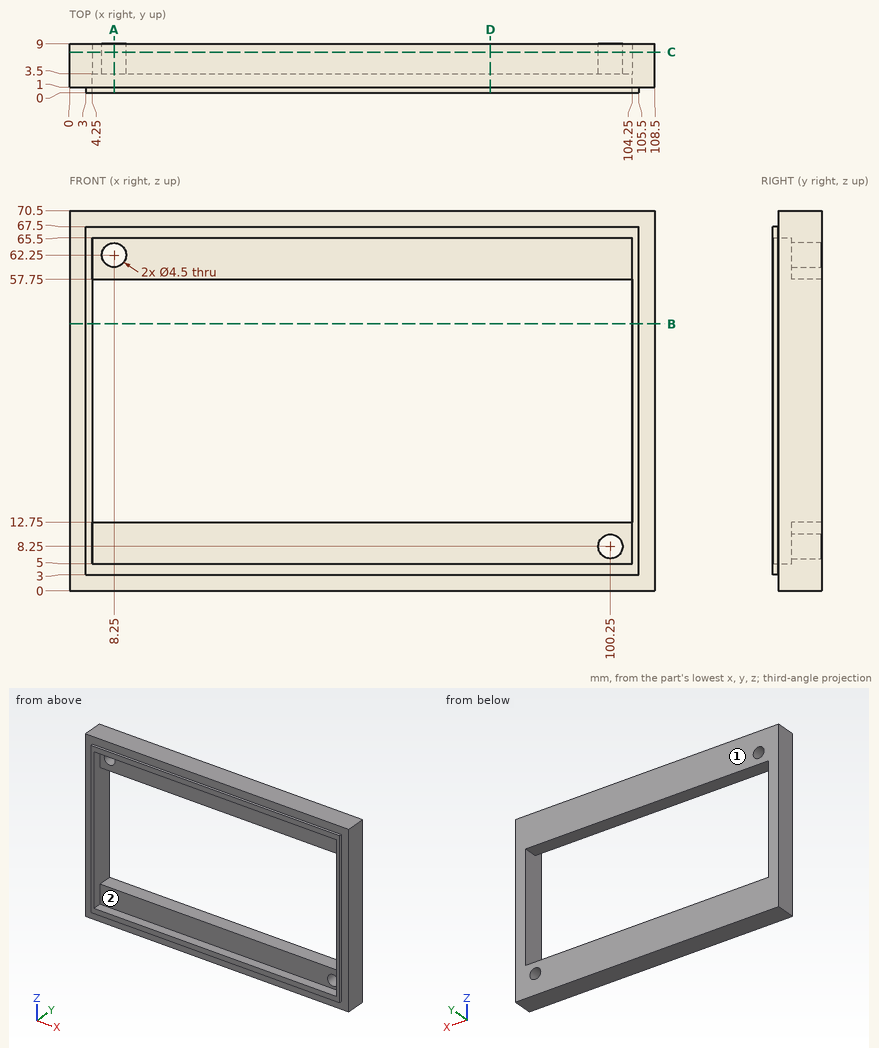
The figure shows three views and two pictorial views of one solid part (mm, origin at its lowest corner). Answer the questions. Coordinates: 2 decimals unless noted, no trailing zeros. Order: outer loops, then holes, each group sorted by start corner. A loop starts at its lowest first (then second) coordinate and runs counter-clockwise, first axis right, second up. Notation, with made-up numbers: (2.25, 30.5) - (44.25, 30.5) arc R30 cw to (44.25, 56.5) - close; hole circle Ø10 at (20, 14). An arc over 180 degrees is marked (long way). Answer as a JSON object with one key per item and string values.
1. Find section D-D on x = 78. Determine the outline of the cut face in (y, z).
Output values:
{"outline": "(0, 3) - (1, 3) - (1, 0) - (9, 0) - (9, 12.75) - (3.5, 12.75) - (3.5, 5) - (0, 5) - close; (0, 65.5) - (3.5, 65.5) - (3.5, 57.75) - (9, 57.75) - (9, 70.5) - (1, 70.5) - (1, 67.5) - (0, 67.5) - close"}
2. Find section C-C on y = 7.5. Determine the outline of the cut face in (x, z).
Output values:
{"outline": "(0, 0) - (108.5, 0) - (108.5, 70.5) - (0, 70.5) - close; hole (4.25, 12.75) - (104.25, 12.75) - (104.25, 57.75) - (4.25, 57.75) - close; hole circle Ø4.5 at (8.25, 62.25); hole circle Ø4.5 at (100.25, 8.25)"}
3. Consider line 1 (Z direction, x = 100.25, y = 7.6); line 2 (X direction, y = 0.75, z = 12); line 3 (Z direction, x = 83.5, y = 2). Determine where each line is inside the solid, lowest interval first.
Output values:
{"line 1": "z = 0 to 6, 10.5 to 12.75, 57.75 to 70.5", "line 2": "x = 3 to 4.25, 104.25 to 105.5", "line 3": "z = 0 to 5, 65.5 to 70.5"}
4. Find section A-A on x = 8.25. Determine the outline of the cut face in (y, z), plus the area to 4 significant figures.
Output values:
{"outline": "(0, 3) - (1, 3) - (1, 0) - (9, 0) - (9, 12.75) - (3.5, 12.75) - (3.5, 5) - (0, 5) - close; (0, 65.5) - (3.5, 65.5) - (3.5, 64.5) - (9, 64.5) - (9, 70.5) - (1, 70.5) - (1, 67.5) - (0, 67.5) - close; (3.5, 57.75) - (9, 57.75) - (9, 60) - (3.5, 60) - close", "area": "144.5 mm²"}
5. Each of these flat-tipped pins is pushed along its axis until it touches: P1, Ø0.5, axis at y = 0.5, z = 29, coming from the -X side; P2, Ø4, axis at x = 72.5, z = 9, coming from the -Y side; P3, Ø0.8, axis at y = 0.5, z = 41, coming from the +X side; P4, Ø4, axis at x = 8.25, z = 62.25, coming from the -Y side. Where does it stop, or does it pass through?
Output values:
{"P1": "stops at x = 3", "P2": "stops at y = 3.5", "P3": "stops at x = 105.5", "P4": "passes through"}
6. The mould has two halves that part along Z. Classify the marked faces 1 and 2: +Z half, -Z half, draft (parallel to the pull), parting line (faces both ways), or undercut.
Output values:
{"face 1": "draft", "face 2": "undercut"}
7. Find section B-B on z = 49.5. Determine the outline of the cut face in (x, y).
Output values:
{"outline": "(0, 1) - (3, 1) - (3, 0) - (4.25, 0) - (4.25, 9) - (0, 9) - close; (104.25, 0) - (105.5, 0) - (105.5, 1) - (108.5, 1) - (108.5, 9) - (104.25, 9) - close"}
